from build123d import *

# Parameters (mm, degrees)
SKETCH_1_W      = 30
SKETCH_1_H      = 49
SKETCH_1_R      = 1
EXTRUDE_1_DEPTH = 1.6
SKETCH_2_W      = 30
SKETCH_2_H      = 38
EXTRUDE_2_DEPTH = 1.5
SKETCH_3_W      = 8.4
SKETCH_3_H      = 5
EXTRUDE_3_DEPTH = 2


with BuildPart() as part:
    # 草图1 → 凸台-拉伸1 (new body)
    with BuildSketch(Plane(origin=(0, 0, 0), x_dir=(1, 0, 0), z_dir=(0, 1, 0))):
        with Locations((15, -24.5)):
            Rectangle(SKETCH_1_W, SKETCH_1_H)
        with BuildLine():
            ThreePointArc((2.8, -47.2), (1.8, -46.2), (2.8, -45.2))
            Line((2.8, -45.2), (10.8, -45.2))
            ThreePointArc((10.8, -45.2), (11.507106781, -45.492893219), (11.8, -46.2))
            ThreePointArc((11.8, -46.2), (11.507106781, -46.907106781), (10.8, -47.2))
            Line((10.8, -47.2), (2.8, -47.2))
        make_face(mode=Mode.SUBTRACT)
        with BuildLine():
            ThreePointArc((19.2, -47.2), (18.2, -46.2), (19.2, -45.2))
            Line((19.2, -45.2), (27.2, -45.2))
            ThreePointArc((27.2, -45.2), (27.907106781, -45.492893219), (28.2, -46.2))
            ThreePointArc((28.2, -46.2), (27.907106781, -46.907106781), (27.2, -47.2))
            Line((27.2, -47.2), (19.2, -47.2))
        make_face(mode=Mode.SUBTRACT)
        with Locations(Location((3, -2.6, 0), (0, 0, 270))):
            Circle(SKETCH_1_R, mode=Mode.SUBTRACT)
        with Locations(Location((27, -2.6, 0), (0, 0, 270))):
            Circle(SKETCH_1_R, mode=Mode.SUBTRACT)
    extrude(amount=EXTRUDE_1_DEPTH)

    # 草图2 → 凸台-拉伸2 (add)
    with BuildSketch(Plane(origin=(0, 1.6, 0), x_dir=(1, 0, 0), z_dir=(0, 1, 0))):
        with Locations((15, -24.7)):
            Rectangle(SKETCH_2_W, SKETCH_2_H)
    extrude(amount=EXTRUDE_2_DEPTH)

    # 草图3 → 凸台-拉伸3 (add)
    with BuildSketch(Plane.XZ):
        with Locations((15, 38)):
            Rectangle(SKETCH_3_W, SKETCH_3_H)
    extrude(amount=EXTRUDE_3_DEPTH)


solid = part.part
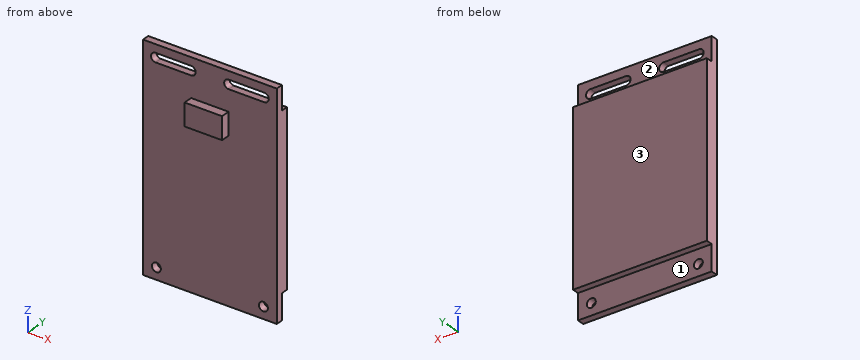
Read the model definition and answer for the solid it produces. Units are mm, in the model's axes. Face numbers are marked on the shaded views. A direction names the side the tool comes from. Coordinates: 2 decimals unless noted, no trailing zeros. Write each loop counter-clockwise with the first axis right and the second up, starting at its lowest first coordinate (ties: lowest second). Pieces come first, ordered by that corner, then holes. Notation, with made-up numbers: M -12.5,21.25 L 6.5,21.25 A25 ccw 6.5,39.25 Z; hole C 0,87.25 d6. An arc over 180 degrees is marked long. Use a Markdown table: item, result.
Q1. The part is cut by section A-A, the plane z = 2.6. Write down the section's boundary in (x, y).
Answer block:
| item | result |
|---|---|
| outline | M 0,0 L 2,0 L 2,1.6 L 0,1.6 Z; M 4,0 L 26,0 L 26,1.6 L 4,1.6 Z; M 28,0 L 30,0 L 30,1.6 L 28,1.6 Z |
Q2. The part is cut by section C-C, the plane z = 39. Write down the section's boundary in (x, y), then the cut area to 3 significant figures.
Answer block:
| item | result |
|---|---|
| outline | M 0,0 L 10.8,0 L 10.8,-2 L 19.2,-2 L 19.2,0 L 30,0 L 30,3.1 L 0,3.1 Z |
| area | 110 mm2 |
Q3. The part is cut by section D-D, the plane z = 8. Write down the section's boundary in (x, y), then the cut area to 3 significant figures.
Answer block:
| item | result |
|---|---|
| outline | M 0,0 L 30,0 L 30,3.1 L 0,3.1 Z |
| area | 93.0 mm2 |
Q4. Which of the six approach directions +Z, -Z, +X, -X, +Y, -Y give full straight-line access (tool end or side, diameter ignored) to the marked faces 1, 2 and 3?
Answer block:
| item | result |
|---|---|
| face 1 | -Z, +X, -X, +Y |
| face 2 | +Z, +X, -X, +Y |
| face 3 | +Z, -Z, +X, -X, +Y |
Q5. Each of these flat-tipped pins is pushed along its axis until it touches: pin 1 Ø3 at (x, z) = (18.5, 2.5) entering from +Y; pin 2 Ø0.8 at (x, y) = (16, 2.5) entering from -Z; pin 3 Ø0.6 at (y, z) = (-1, 37) entering from -X. Where does it stop, or does it pass through?
Answer block:
| item | result |
|---|---|
| pin 1 | stops at y = 1.6 |
| pin 2 | stops at z = 5.7 |
| pin 3 | stops at x = 10.8 |
Q6. Straight lines are drawn through the part: L1, parallel to X at y = 1, z = 2.6; L2, parallel to Y at x = 6.5, z = 40; L3, parallel to Z at x = 11.75, y = 1.95. For each, find the intervals that lie inside material, in ascending order. Write a range as [from, to].
Answer block:
| item | result |
|---|---|
| L1 | x = [0, 2], [4, 26], [28, 30] |
| L2 | y = [0, 3.1] |
| L3 | z = [5.7, 43.7] |
Q7. The part is cut by section B-B, the plane x = 22. Write down the section's boundary in (y, z), then the cut area to 3 significant figures.
Answer block:
| item | result |
|---|---|
| outline | M 0,0 L 1.6,0 L 1.6,5.7 L 3.1,5.7 L 3.1,43.7 L 1.6,43.7 L 1.6,45.2 L 0,45.2 Z; M 0,47.2 L 1.6,47.2 L 1.6,49 L 0,49 Z |
| area | 132 mm2 |
